Can you work these out from the model? Positions are in its coordinate system, mm. Give positions to 0.01 mm unless a question says otherwise; leave off trailing zeros. Order: outer loops, then holes, each group sorted by start corner. A loop starts at its lowest first (then second) coordinate and runs counter-clockwise, first axis right, second up. Notation, with made-up numbers: M 46,82 L 55,82 A26 cw 55,109 Z; hole C 6,34.25 d4. An arc over 180 degrees is marked long. Write each question's results on one line, items separated by ' | '.
from build123d import *

# Parameters (mm, degrees)
EXTRUDE_1_DEPTH     = 2
SKETCH_2_W          = 48
SKETCH_2_H          = 50.191121785
CUT_EXTRUDE_1_DEPTH = 10
SKETCH_3_R          = 2.275
CUT_EXTRUDE_2_DEPTH = 10


with BuildPart() as part:
    # 草图1 → 凸台-拉伸1 (new body)
    with BuildSketch(Plane(origin=(0, 0, 0), x_dir=(1, 0, 0), z_dir=(0, 1, 0))):
        Polygon((-76.5, 42.382061447), (0, 106.573183232), (76.5, 42.382061447), (76.5, -42.382061447), (-76.5, -42.382061447), align=None)
    extrude(amount=EXTRUDE_1_DEPTH)

    # 草图2 → 切除-拉伸1 (cut)
    with BuildSketch(Plane(origin=(0, 2, 0), x_dir=(1, 0, 0), z_dir=(0, 1, 0))):
        with Locations((0, 81.47762234)):
            Rectangle(SKETCH_2_W, SKETCH_2_H)
    extrude(amount=-CUT_EXTRUDE_1_DEPTH, mode=Mode.SUBTRACT)

    # 草图3 → 切除-拉伸2 (cut)
    with BuildSketch(Plane(origin=(0, 2, 0), x_dir=(1, 0, 0), z_dir=(0, 1, 0))):
        with Locations(Location((14, 52.382061447, 0), (0, 0, 270))):
            Circle(SKETCH_3_R)
        with Locations(Location((-14, 52.382061447, 0), (0, 0, 270))):
            Circle(SKETCH_3_R)
    extrude(amount=-CUT_EXTRUDE_2_DEPTH, mode=Mode.SUBTRACT)


solid = part.part
(1) Imagine slicing it at B-B, the plane x = -14. Write out the boundary of the cut face in (y, z), plus the area to 3 significant figures.
Data:
outline: M 0,-56.38 L 2,-56.38 L 2,-54.66 L 0,-54.66 Z; M 0,-50.11 L 2,-50.11 L 2,42.38 L 0,42.38 Z | area: 188 mm2
(2) We'd pull the mould along X, two halves only. Please class faces 1 (the face through (49.9, 1, -64.7)), 2 (the face through (-12.08, 1.01, -51.16)), 3 (the face through (-50.62, 0.99, -64.1)): +X half, -X half, draft (parallel to the pull), parting line (faces both ways), or undercut.
Data:
face 1: +X half | face 2: undercut | face 3: -X half
(3) Imagine slicing it at D-D, the plane z = -44.5. Write out the boundary of the cut face in (x, y), plus the area to 3 significant figures.
Data:
outline: M -73.98,0 L 73.98,0 L 73.98,2 L -73.98,2 Z | area: 296 mm2
(4) Imagine slicing it at A-A, the plane y = 1.7. Write out the boundary of the cut face in (x, z) (3 decimals), plus the area to 3 significant figures.
Data:
outline: M -76.5,-42.382 L -24,-86.435 L -24,-56.382 L 24,-56.382 L 24,-86.435 L 76.5,-42.382 L 76.5,42.382 L -76.5,42.382 Z; hole C -14,-52.382 d4.55; hole C 14,-52.382 d4.55 | area: 15,900 mm2
(5) I need wall thicknesses on L1, parallel to X at y = 1.7, z = -50.5; L2, parallel to X at y = 0.1, z = -70; L3, parallel to X at y = 0.6, z = -58. Which ranges of each line are inside material? Lowest first, please. Write a range as from..to.
Data:
L1: x = -66.83..-15.28, -12.72..12.72, 15.28..66.83 | L2: x = -43.59..-24, 24..43.59 | L3: x = -57.89..-24, 24..57.89
(6) Will this pin go through, and if not, where does the flat tip stop? P1, Ø8, axis at x = 56.5, z = -39.5, coming from the -Y side.
Data:
P1: stops at y = 0
(7) Imagine slicing it at C-C, the plane x = 7. Write out the boundary of the cut face in (y, z), plus the area to 3 significant figures.
Data:
outline: M 0,-56.38 L 2,-56.38 L 2,42.38 L 0,42.38 Z | area: 198 mm2
